Work out the finished part from the listing and answer in its coordinate system (mm). Face numbers are marked on the shaded views. A direction names the side the tool comes from. Give positions to 0.01 mm unless a question says otherwise; leave off trailing zeros. Loops run counter-clockwise (first coordinate to the right, second up) from the corner with the lowest first, then second, coordinate; pieces in that order, holes last. Notation, with made-up numbers: M 45.5,50.5 L 49.5,50.5 A21 ccw 49.5,76.5 Z; hole C -5,53.5 d8. An arc over 180 degrees is marked long. Write item = value, one per line. Start each with the question number.
1. Section B-B on x = 201 is taken. Determine the outline of the cut face in (y, z) (1 decimal), plus the area to 3 significant figures.
2. Flat-ended cylindrical pins translate along their axes: pin 1 Ø5 at (x, y) = (-179, -51.5) entering from +Z; pin 2 Ø10 at (x, z) = (-159.5, -12) entering from +Y; pin 3 Ø12 at (y, z) = (-60, -118) entering from -X; pin 4 Ø23 at (y, z) = (-66.16, 141.07) entering from +X. Find the tip coordinate at first contact, or state that the pin passes through.
3. For the marked faces 1 and 2, determine the directions among +Z, -Z, +X, -X, +Y, -Y from which every point of the face is accessible in a straight line to the end or side of a thin tool.
4. Section A-A on y = 110 is taken. Determine the outline of the cut face in (x, z), plus the area to 3 significant figures.
5. Consider L1, parallel to X at y = 55.5, z = -127; L2, parallel to Z at x = 303, y = 33.5; L3, parallel to X at y = -20, z = 74. Determine where each line is inside the solid, lowest interval first. Write a range as [from, to].
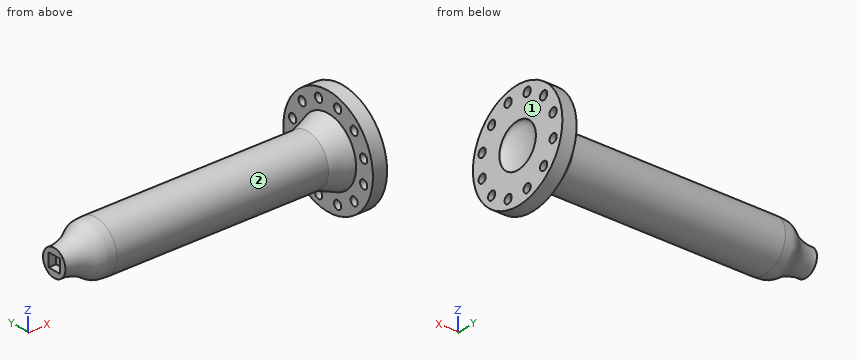
```python
from build123d import *

# Parameters (mm, degrees)
F0_W     = 711.2
F0_H     = 84.1375
F2_W     = 44.45
F2_H     = 44.45
F3_DEPTH = 25.4
F4_R     = 14.2875
F5_DEPTH = 968.2490001


with BuildPart() as f1:
    # F0 (on Top) → F1 (revolve)
    with BuildSketch(Plane.XY):
        with BuildLine():
            Line((-355.6, -28.3585746473), (-355.6, 55.7789253527))
            add(Edge.make_bspline(
                [(-495.3, 16.0914253527), (-491.1825215885, 15.7318338139), (-479.4418370711, 14.7064851925), (-427.3573599541, 26.8287985997), (-400.0577825465, 54.9384491614), (-370.6219245107, 55.4949352575), (-355.6, 55.7789253527)],
                knots=[0, 0, 0, 0, 0.1628231526, 0.4642781518, 0.7266064691, 1, 1, 1, 1], degree=3))
            Line((-495.3, 16.0914253527), (-495.3, -28.3585746473))
            Line((-495.3, -28.3585746473), (-355.6, -28.3585746473))
        make_face()
        with Locations((0, 13.7101753527)):
            Rectangle(F0_W, F0_H)
        with BuildLine():
            Line((425.196, 82.7664253527), (355.6, 55.7789253527))
            Line((355.6, 55.7789253527), (355.6, -28.3585746473))
            Line((355.6, -28.3585746473), (451.6144843253, -28.3585746473))
            add(Edge.make_bspline(
                [(472.948, 44.1196709871), (451.6144843253, 44.1196709871), (451.6144843253, -28.3585746473)],
                knots=[0, 0, 0, 1.5707963268, 1.5707963268, 1.5707963268], degree=2, weights=[1, 0.7071067812, 1]))
            Line((472.948, 44.1196709871), (472.948, 149.4414253527))
            Line((472.948, 149.4414253527), (425.196, 149.4414253527))
            Line((425.196, 149.4414253527), (425.196, 82.7664253527))
        make_face()
    revolve(axis=Axis((-425.45, -28.3585746473, 0), (-1, 0, 0)))

    # F2 (on face) → F3 (cut)
    with BuildSketch(Plane(origin=(-495.3, 0, 0), x_dir=(0, -1, 0), z_dir=(-1, 0, 0))):
        with Locations((28.3585746473, 0)):
            Rectangle(F2_W, F2_H)
    extrude(amount=-F3_DEPTH, mode=Mode.SUBTRACT)

    # F4 (on face) → F5 (cut, through all)
    with BuildSketch(Plane.YZ.offset(472.948)):
        with Locations((-131.6315200396, 103.2729453923)):
            Circle(F4_R)
        with Locations((-66.1590961845, 141.0734669295)):
            Circle(F4_R)
        with Locations((9.4419468899, 141.0734669295)):
            Circle(F4_R)
        with Locations((74.914370745, 103.2729453923)):
            Circle(F4_R)
        with Locations((112.7148922822, 37.8005215372)):
            Circle(F4_R)
        with Locations((112.7148922822, -37.8005215372)):
            Circle(F4_R)
        with Locations((74.914370745, -103.2729453923)):
            Circle(F4_R)
        with Locations((9.4419468899, -141.0734669295)):
            Circle(F4_R)
        with Locations((-66.1590961845, -141.0734669295)):
            Circle(F4_R)
        with Locations((-131.6315200396, -103.2729453923)):
            Circle(F4_R)
        with Locations((-169.4320415768, -37.8005215372)):
            Circle(F4_R)
        with Locations((-169.4320415768, 37.8005215372)):
            Circle(F4_R)
    extrude(amount=-F5_DEPTH, mode=Mode.SUBTRACT)


solid = f1.part
```
Verdict:
q1.outline = C -28.4,0 d168.3
q1.area = 22,200 mm2
q2.pin_1 = 81.57
q2.pin_2 = 55.49
q2.pin_3 = 425.2
q2.pin_4 = through
q3.face_1 = +Z, -Z, +X, +Y, -Y
q3.face_2 = -X
q4.outline = M 425.2,-111.67 L 472.95,-111.67 L 472.95,-51.83 L 425.2,-51.83 Z; M 425.2,-23.77 L 472.95,-23.77 L 472.95,23.77 L 425.2,23.77 Z; M 425.2,51.83 L 472.95,51.83 L 472.95,111.67 L 425.2,111.67 Z
q4.area = 7,990 mm2
q5.L1 = [425.2, 472.95]
q5.L2 = [-57.03, 57.03]
q5.L3 = [-405.89, 472.95]
